```python
from build123d import *

# Parameters (mm, degrees)
SKETCH1_R            = 9.525
BOSS_EXTRUDE1_DEPTH  = 12.7
SKETCH9_R            = 17.4625
BOSS_EXTRUDE2_DEPTH  = 4.7625
SKETCH2_R            = 4.572
CUT_EXTRUDE1_DEPTH   = 2.9972
M2_CLEARANCE_HOLE1_D = 2.4
SKETCH6_R            = 1.9
CUT_EXTRUDE2_DEPTH   = 2.54
SKETCH7_R            = 1.499997
CUT_EXTRUDE3_DEPTH   = 28.769908399
CIRPATTERN1_COUNT    = 3
CIRPATTERN2_COUNT    = 3
FILLET1_R            = 1.5875


with BuildPart() as part:
    # Sketch1 → Boss-Extrude1 (new body)
    with BuildSketch(Plane.XY):
        Circle(SKETCH1_R)
    extrude(amount=BOSS_EXTRUDE1_DEPTH)

    # Sketch9 → Boss-Extrude2 (add)
    with BuildSketch(Plane.XY.offset(12.7)):
        Circle(SKETCH9_R)
    extrude(amount=-BOSS_EXTRUDE2_DEPTH)

    # Sketch2 → Cut-Extrude1 (cut)
    with BuildSketch(Plane(origin=(0, 0, 0), x_dir=(-1, 0, 0), z_dir=(0, 0, -1))):
        Circle(SKETCH2_R)
    extrude(amount=-CUT_EXTRUDE1_DEPTH, mode=Mode.SUBTRACT)

    # M2 Clearance Hole1 (through all)
    with Locations(Plane(origin=(0, 0, 0), x_dir=(-1, 0, 0), z_dir=(0, 0, -1))):
        with Locations((0, 6.0000007)):
            m2_clearance_hole1 = Hole(M2_CLEARANCE_HOLE1_D / 2)

    # Sketch6 → Cut-Extrude2 (cut)
    with BuildSketch(Plane.XY.offset(12.7)):
        with Locations((0, 6.0000007)):
            Circle(SKETCH6_R)
    cut_extrude2 = extrude(amount=-CUT_EXTRUDE2_DEPTH, mode=Mode.SUBTRACT)

    # Sketch7 → Cut-Extrude3 (cut, through all)
    with BuildSketch(Plane(origin=(0, 0, 0), x_dir=(-1, 0, 0), z_dir=(0, 0, -1))):
        with Locations((12.373337957, 7.14375)):
            Circle(SKETCH7_R)
    cut_extrude3 = extrude(amount=-CUT_EXTRUDE3_DEPTH, mode=Mode.SUBTRACT)

    # CirPattern1: M2 Clearance Hole1, Cut-Extrude2 ×3 about axis
    cirpattern1_axis = Axis((0, 0, 0), (0, 0, 1))
    add([m2_clearance_hole1.rotate(cirpattern1_axis, i * 360 / CIRPATTERN1_COUNT) for i in range(1, CIRPATTERN1_COUNT)], mode=Mode.SUBTRACT)
    add([cut_extrude2.rotate(cirpattern1_axis, i * 360 / CIRPATTERN1_COUNT) for i in range(1, CIRPATTERN1_COUNT)], mode=Mode.SUBTRACT)

    # CirPattern2: Cut-Extrude3 ×3 about axis
    cirpattern2_axis = Axis((0, 0, 0), (0, 0, 1))
    for i in range(1, CIRPATTERN2_COUNT):
        add(cut_extrude3.rotate(cirpattern2_axis, i * 360 / CIRPATTERN2_COUNT), mode=Mode.SUBTRACT)

    # Fillet1
    fillet1_edges = [part.edges().sort_by_distance(p)[0] for p in [
        (-9.525, 0, 7.9375),
    ]]
    fillet(fillet1_edges, radius=FILLET1_R)


solid = part.part
```
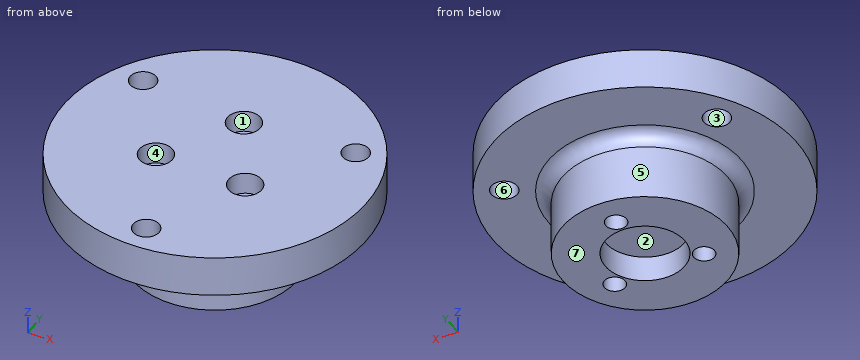
Check sheet for the modelled part. Datum: model origin and axes. Units: mm. Face numbers are marked on the shaded views. A direction names the side the tool comes from. Round coordinates to 2 decimals unless told otherwise and drop trailing zeros.
1) Section check A-A (x = 0). Give the number of separate pieces and of enclosed holes in the cut face, and give its area (3 significant figures).
2) Go/stop test with flat-tipped pins: pin 1 Ø1.9 at (x, y) = (5, -3.5) entering from +Z; pin 2 Ø8 at (x, y) = (-6, -7) entering from -Z; pin 3 Ø5 at (x, y) = (12.37, 7.14) entering from -Z; pin 4 Ø6 at (x, z) = (7, 6.5) entering from +Y. Record where each tip stops, or that it passes through.
3) Scan lines: line 1 (Y direction, x = 0, z = 10); line 2 (X direction, y = -3, z = 11.3); line 3 (X direction, y = -3, z = 3.75). Record each from-to range of solid material in increasing order.
4) Mould release check, pull along X, two halves, no side actions. Record for the marked faces 4, 5, 6 and 7: +X half, -X half, draft (parallel to the pull), parting line (faces both ways), or undercut.
5) Tool access check on the marked faces 1, 2 and 3. Record the directions out of +Z, -Z, +X, -X, +Y, -Y that give a thin tool (end or side, any length) a straight path to the whole face; none if there is none.
Result:
1. separate pieces: 3
1. enclosed holes: 0
1. area: 243 mm2
2. pin 1: stops at z = 10.16
2. pin 2: stops at z = 0
2. pin 3: stops at z = 7.94
2. pin 4: stops at y = 16.91
3. line 1: y = -17.46 to -15.79, -12.79 to 4.8, 7.2 to 17.46
3. line 2: x = -17.2 to -7.1, -3.3 to 3.3, 7.1 to 17.2
3. line 3: x = -9.04 to -6.4, -4 to 4, 6.4 to 9.04
4. face 4: undercut
4. face 5: parting line
4. face 6: undercut
4. face 7: draft
5. face 1: +Z
5. face 2: -Z
5. face 3: +Z, -Z
